Here's how the part is built. I have some questions about the finished solid (model axes, mm). Give positions to 0.01 mm unless a question says otherwise; leave off trailing zeros. Loops run counter-clockwise (first coordinate to the right, second up) from the corner with the lowest first, then second, coordinate; pieces in that order, holes last. Notation, with made-up numbers: M 12,57 L 68,57 A5 cw 68,61 Z; hole C 67,68.5 d5. An arc over 180 degrees is marked long. Answer as CSV lines item,"result". Start each with the question number.
Item 1: I want a section at B-B on x = -4. List the corners of the cut face in (y, z) for me, plus the area to 3 significant figures.
Item 2: Will these pins go through, and if not, where does the flat tip stop? P1, Ø1.5, axis at y = -2, z = 6, coming from the +X side; P2, Ø1, axis at x = 17.5, y = -0.5, coming from the -Z side; P3, Ø1, axis at y = -0.5, z = 0.5, coming from the -X side.
Item 3: I want a section at A-A on x = 25. List the corners of the cut face in (y, z) for me.
Item 4: I want a section at D-D on z = 0. List the corners of the cut face in (x, y) for me, plus the area to 3 significant figures.
Item 5: I want a section at C-C on y = -1.9. List the corners of the cut face in (x, z) for me.
Item 6: If I drill on line 1 along Z through (x, y) = (0, -1.3); line 2 along Z through (x, y) = (3, -2.2); line 3 along Z through (x, y) = (14.5, -0.6), over which ranges is the centre line in solid material (lowest first)? Write a range as from..to.
from build123d import *

# Parameters (mm, degrees)
F1_DEPTH = 3


with BuildPart() as f1:
    # F0 (on Front) → F1 (new body)
    with BuildSketch(Plane.XZ):
        with BuildLine():
            ThreePointArc((-23.9565223957, 19.6744767327), (10.4486316265, 29.1860599796), (31, 0))
            ThreePointArc((31, 0), (21.9203102168, -21.9203102168), (0, -31))
            ThreePointArc((0, -31), (3.7951823528, -31.5663122562), (7.2597095854, -33.2159090909))
            ThreePointArc((7.2597095854, -33.2159090909), (26.4842417855, -21.3209975622), (34, 0))
            ThreePointArc((34, 0), (11.4597895259, 32.010517397), (-26.2748955308, 21.578458352))
            Line((-26.2748955308, 21.578458352), (-23.9565223957, 19.6744767327))
        make_face()
        with BuildLine():
            ThreePointArc((7.2597095854, -33.2159090909), (3.7951823528, -31.5663122562), (0, -31))
            ThreePointArc((0, -31), (-3.7951823528, -31.5663122562), (-7.2597095854, -33.2159090909))
            ThreePointArc((-7.2597095854, -33.2159090909), (-3.6509650286, -33.8034089163), (-5.1e-08, -34))
            ThreePointArc((-5.1e-08, -34), (3.6509649778, -33.8034089217), (7.2597095854, -33.2159090909))
        make_face()
        with BuildLine():
            ThreePointArc((-5.1e-08, -34), (-3.6509650286, -33.8034089163), (-7.2597095854, -33.2159090909))
            ThreePointArc((-7.2597095854, -33.2159090909), (-6.1083457413, -55.4755440963), (13, -44))
            Line((13, -44), (10, -44))
            ThreePointArc((10, -44), (-7.0710677938, -51.0710678299), (-5.1e-08, -34))
        make_face()
    extrude(amount=F1_DEPTH)


solid = f1.part
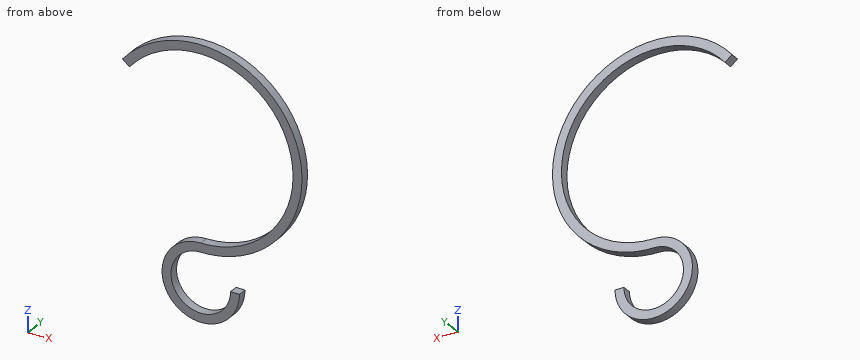
Result:
1,outline,"M -3,-56.37 L 0,-56.37 L 0,-53.17 L -3,-53.17 Z; M -3,-34.83 L 0,-34.83 L 0,-31.63 L -3,-31.63 Z; M -3,30.74 L 0,30.74 L 0,33.76 L -3,33.76 Z"
1,area,"28.3 mm^2"
2,P1,"x = 33.59"
2,P2,"z = -29.44"
2,P3,"x = 30.98"
3,outline,"M -3,-23.04 L 0,-23.04 L 0,-18.33 L -3,-18.33 Z; M -3,18.33 L 0,18.33 L 0,23.04 L -3,23.04 Z"
4,outline,"M 31,-3 L 34,-3 L 34,0 L 31,0 Z"
4,area,"9.00 mm^2"
5,outline,"M -26.27,21.58 L -23.96,19.67 A31 cw long 0,-31 A13 ccw long 13,-44 L 10,-44 A10 cw long 0,-34 A34 ccw long Z"
6,line 1,"-57..-54, -34..-31, 31..34"
6,line 2,"-56.65..-53.54, -33.87..-30.85, 30.85..33.87"
6,line 3,"-30.75..-27.4, 27.4..30.75"
